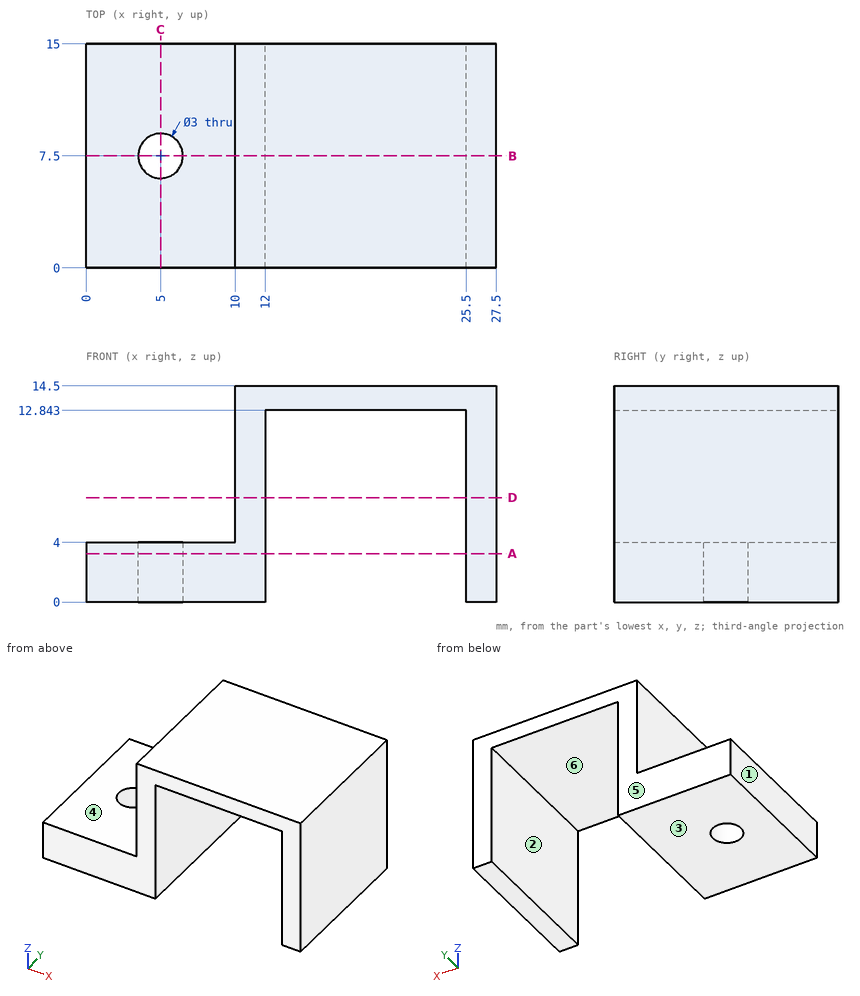
The drawing under review shows one solid part. Ordinate dimensions are in mm from its lowest x, y, z. A direction names the side the tool comes from. Coordinates: 2 decimals unless noted, no trailing zeros. Order: outer loops, then holes, each group sorted by start corner. A loop starts at its lowest first (then second) coordinate and runs counter-clockwise, first axis right, second up. Notation, with made-up numbers: (79.5, 16.25) -> (128.5, 16.25) arc R3 ccw to (128.5, 21.25) -> close; hole circle Ø1 at (15.25, -11.5). An arc over 180 degrees is marked (long way). Answer in a Markdown table with one row per item. Add a question column.
Item 1: We need section A-A on z = 3.25. Write out the cut boundary in (x, y), plus the area to 3 significant figures.
Item 2: To check wall thickness, follow probe 1 along Y at (x, z) = (5, 2.3); probe 2 along X at (y, z) = (11.5, 11.75); probe 3 along X at (y, z) = (5, 1.75). State the ranges of each line that lie inside material, in increasing order.
Item 3: Machinability: for the marked faces 4, 5 and 6, which of the approach directions +Z, -Z, +X, -X, +Y, -Y give a long, thin tool a straight path to every point of the face, cutting with its end or side? Answer none if there is none.
Item 4: We need section B-B on y = 7.5. Write out the cut boundary in (x, z), plus the area to 3 significant figures.
Item 5: We need section C-C on x = 5. Write out the cut boundary in (y, z).
Item 6: Mouldability with a two-part tool opening along X and no side actions: class the marked faces 1, 2 and 3 as +X half, -X half, draft (parallel to the pull), parting line (faces both ways), or undercut.
Item 7: Clearance check with flat-ended pins moving along their axes: pin 1 (4 mm diameter, centred on y = 9, z = 8.5, fed in from -X); pin 2 (5 mm diameter, centred on x = 6, z = 9.5, fed in from +Y); pin 3 (5 mm diameter, centred on x = 4.5, y = 9.5, fed in from +Z); pin 4 (7 mm diameter, centred on x = 20, y = 9, fed in from -Z). State where each tip first meets the part, or that it passes through.
Item 8: We need section D-D on z = 7. Write out the cut boundary in (x, y), plus the area to 3 significant figures.
Final values:
| question | item | result |
|---|---|---|
| 1 | outline | (0, 0) -> (12, 0) -> (12, 15) -> (0, 15) -> close; (25.5, 0) -> (27.5, 0) -> (27.5, 15) -> (25.5, 15) -> close; hole circle Ø3 at (5, 7.5) |
| 1 | area | 203 mm2 |
| 2 | probe 1 | y = 0 to 6, 9 to 15 |
| 2 | probe 2 | x = 10 to 12, 25.5 to 27.5 |
| 2 | probe 3 | x = 0 to 12, 25.5 to 27.5 |
| 3 | face 4 | +Z, -X, +Y, -Y |
| 3 | face 5 | +Z, -Z, +X, -X, +Y |
| 3 | face 6 | -Z, +Y, -Y |
| 4 | outline | (0, 0) -> (3.5, 0) -> (3.5, 4) -> (0, 4) -> close; (6.5, 0) -> (12, 0) -> (12, 12.84) -> (25.5, 12.84) -> (25.5, 0) -> (27.5, 0) -> (27.5, 14.5) -> (10, 14.5) -> (10, 4) -> (6.5, 4) -> close |
| 4 | area | 108 mm2 |
| 5 | outline | (0, 0) -> (6, 0) -> (6, 4) -> (0, 4) -> close; (9, 0) -> (15, 0) -> (15, 4) -> (9, 4) -> close |
| 6 | face 1 | -X half |
| 6 | face 2 | undercut |
| 6 | face 3 | draft |
| 7 | pin 1 | stops at x = 10 |
| 7 | pin 2 | passes through |
| 7 | pin 3 | stops at z = 4 |
| 7 | pin 4 | stops at z = 12.84 |
| 8 | outline | (10, 0) -> (12, 0) -> (12, 15) -> (10, 15) -> close; (25.5, 0) -> (27.5, 0) -> (27.5, 15) -> (25.5, 15) -> close |
| 8 | area | 60.0 mm2 |
